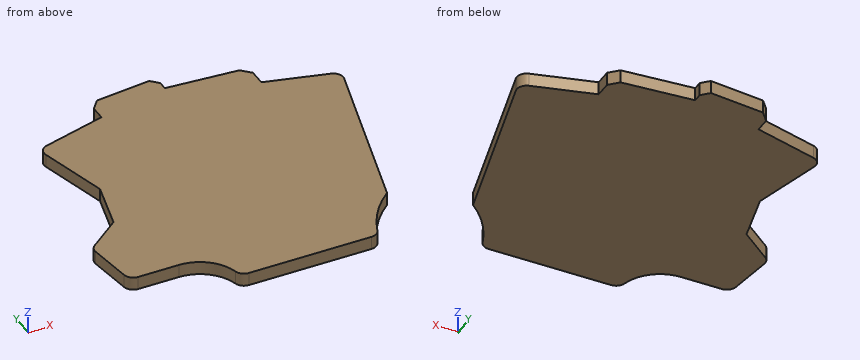
```python
from build123d import *

# Parameters (mm, degrees)
BOSS_EXTRUDE2_DEPTH   = 4
FILLET3_R             = 3
CHAMFER1_SIZE2        = 2.5
CHAMFER1_SIZE         = 2.808402332
CHAMFER1_EDGE_2_SIZE2 = 2.5
CHAMFER1_EDGE_2_SIZE  = 2.275013623
CHAMFER1_EDGE_3_SIZE2 = 2.5
CHAMFER1_EDGE_3_SIZE  = 2.72195283


with BuildPart() as part:
    # Sketch1 → Boss-Extrude2 (new body)
    with BuildSketch(Plane.XY):
        with BuildLine():
            ThreePointArc((-159.244638184, -33.673282531), (-150.584384146, -37.159404343), (-146.754642187, -45.673282531))
            Line((-146.754642187, -45.673282531), (-104.73463418, -45.673282531))
            ThreePointArc((-104.73463418, -45.673282531), (-100.473058927, -36.575080639), (-93.705391257, -29.149653001))
            Line((-93.705391257, -29.149653001), (-78.674501487, 26.946391303))
            Line((-78.674501487, 26.946391303), (-100.174501487, 32.70729894))
            Line((-100.174501487, 32.70729894), (-100.174501487, 40.20729894))
            Line((-100.174501487, 40.20729894), (-124.674501487, 42.135490757))
            Line((-124.674501487, 42.135490757), (-124.674501487, 47.335490757))
            Line((-124.674501487, 47.335490757), (-146.174501487, 45.079555506))
            Line((-146.174501487, 45.079555506), (-146.174501487, 37.779555506))
            Line((-146.174501487, 37.779555506), (-168.390795492, 31.826717469))
            Line((-168.390795492, 31.826717469), (-161.960014873, 7.826717469))
            Line((-161.960014873, 7.826717469), (-165.824598917, -7.673282531))
            Line((-165.824598917, -7.673282531), (-176.704102791, -16.173282531))
            Line((-176.704102791, -16.173282531), (-174.244638184, -33.673282531))
            Line((-174.244638184, -33.673282531), (-159.244638184, -33.673282531))
        make_face()
    extrude(amount=BOSS_EXTRUDE2_DEPTH)

    # Fillet3
    fillet3_edges = [part.edges().sort_by_distance(p)[0] for p in [
        (-104.73463418, -45.673282531, 2),
        (-146.754642187, -45.673282531, 2),
        (-174.244638184, -33.673282531, 2),
        (-176.704102791, -16.173282531, 2),
        (-168.390795492, 31.826717469, 2),
        (-78.674501487, 26.946391303, 2),
    ]]
    fillet(fillet3_edges, radius=FILLET3_R)

    # Chamfer1
    chamfer1_edges = [part.edges().sort_by_distance(p)[0] for p in [
        (-146.174501487, 45.079555506, 2),
    ]]
    chamfer(chamfer1_edges, length=CHAMFER1_SIZE, length2=CHAMFER1_SIZE2)

    # Chamfer1 edge 2
    chamfer1_edge_2_edges = [part.edges().sort_by_distance(p)[0] for p in [
        (-124.674501487, 47.335490757, 2),
    ]]
    chamfer(chamfer1_edge_2_edges, length=CHAMFER1_EDGE_2_SIZE, length2=CHAMFER1_EDGE_2_SIZE2)

    # Chamfer1 edge 3
    chamfer1_edge_3_edges = [part.edges().sort_by_distance(p)[0] for p in [
        (-100.174501487, 40.20729894, 2),
    ]]
    chamfer(chamfer1_edge_3_edges, length=CHAMFER1_EDGE_3_SIZE, length2=CHAMFER1_EDGE_3_SIZE2)


solid = part.part
```
Work out the finished part from the listing and answer in its coordinate system (mm). Give positions to 0.01 mm unless a question says otherwise; leave off trailing zeros. Write each loop counter-clockwise with the first axis right and the second up, starting at its lowest first coordinate (ties: lowest second). Pieces come first, ordered by that corner, then holes.
(1) The part is cut by section C-C on x = -142. Write down the section's boundary in (y, z), plus the area to 3 significant figures.
Final values:
outline: (-45.67, 0) - (45.52, 0) - (45.52, 4) - (-45.67, 4) - close
area: 365 mm2
(2) The part is cut by section A-A on z = 1.05. Write down the section's boundary in (x, y).
Final values:
outline: (-176.46, -17.89) - (-174.61, -31.09) arc R3 ccw to (-171.64, -33.67) - (-159.24, -33.67) arc R12.5 cw to (-147.07, -43.35) arc R3 ccw to (-144.14, -45.67) - (-106.9, -45.67) arc R3 ccw to (-104.08, -43.7) arc R33.5 cw to (-93.71, -29.15) - (-79.45, 24.05) arc R3 ccw to (-81.57, 27.72) - (-100.17, 32.71) - (-100.17, 37.71) - (-102.89, 40.42) - (-124.67, 42.14) - (-124.67, 44.84) - (-126.94, 47.1) - (-143.69, 45.34) - (-146.17, 42.27) - (-146.17, 37.78) - (-165.49, 32.6) arc R3 ccw to (-167.61, 28.93) - (-161.96, 7.83) - (-165.82, -7.67) - (-175.34, -15.11) arc R3 ccw to start
(3) The part is cut by section B-B on y = -4. Write down the section's boundary in (x, z).
Final values:
outline: (-164.91, 0) - (-86.97, 0) - (-86.97, 4) - (-164.91, 4) - close
(4) Straight lines are drawn through the part: line 1 (Y direction, x = -124, z = 3.4); line 2 (X direction, y = 25, z = 2.15); line 3 (X direction, y = 8.5, z = 3.3). For each, find the intervals that lie inside material, in ascending order.
Final values:
line 1: y = -45.67 to 42.08
line 2: x = -166.56 to -79.35
line 3: x = -162.14 to -83.62
(5) Flat-ended cylindrical pins translate along their axes: pin 1 Ø1.5 at (x, z) = (-105, 3.5) entering from -Y; pin 2 Ø2 at (y, z) = (35.5, 1) entering from +X; pin 3 Ø1.2 at (x, z) = (-163.5, 3) entering from -Y. Find the tip coordinate at first contact, or state that the pin passes through.
Final values:
pin 1: stops at y = -45.44
pin 2: stops at x = -100.17
pin 3: stops at y = -33.67
